Could you check a few things on this model? Use its own coordinates, in mm. A direction names the side the tool comes from. Coordinates: 2 decimals unless noted, no trailing zeros. Loops run counter-clockwise (first coordinate to the right, second up) from the corner with the lowest first, then second, coordinate; pieces in that order, holes last. Notation, with made-up numbers: M 74,5 L 79,5 A13 cw 79,19 Z; hole C 7.5,3.5 d6. An arc over 180 degrees is marked long. Write each question's results on one line, items separated by ' | '.
```python
from build123d import *

# Parameters (mm, degrees)
SKETCH_1_R                              = 38
SKETCH_1_R_2                            = 36
EXTRUDE_310_DEPTH                       = 15
EXTRUDE_START                           = -9
EXTRUDE_4_DEPTH                         = 9
FILLET_3_RADIUS                         = 5
FILLET_3_LENGTH                         = 9
PATTERN_CIRCULAR_4_COUNT                = 3
FILLET_3_OF_PATTERN_CIRCULAR_4_2_RADIUS = 5
FILLET_3_OF_PATTERN_CIRCULAR_4_2_LENGTH = 9
FILLET_3_OF_PATTERN_CIRCULAR_4_3_RADIUS = 5
FILLET_3_OF_PATTERN_CIRCULAR_4_3_LENGTH = 9
SKETCH_6_W                              = 176.950469939
SKETCH_6_H                              = 123.439451547
CUT_REVOLVE_861_ANGLE                   = 5
SKETCH_14_W                             = 84.084463922
SKETCH_14_H                             = 246.249240822
MM_7_D                                  = 5.2
MM_7_ON_FACE_2_D                        = 5.2
MM_7_ON_FACE_3_D                        = 5.2


with BuildPart() as part:
    # 草图1 → Extrude 310 (new body)
    with BuildSketch(Plane.XY):
        Circle(SKETCH_1_R)
        Circle(SKETCH_1_R_2, mode=Mode.SUBTRACT)
    extrude(amount=EXTRUDE_310_DEPTH)

    # 草图11 → 凸台-拉伸4 (add)
    with BuildSketch(Plane.XY.offset(15).offset(EXTRUDE_START)):
        with BuildLine():
            Line((-5, -37.669616404), (-5, -46.669616404))
            Line((-5, -46.669616404), (5, -46.669616404))
            Line((5, -46.669616404), (5, -37.669616404))
            ThreePointArc((5, -37.669616404), (0, -38), (-5, -37.669616404))
        make_face()
    extrude_4 = extrude(amount=EXTRUDE_4_DEPTH)

    # 圆角3: full round fillet: the end face becomes a half cylinder, R = half its width
    fillet_3_face = Plane((0, -46.669616404, 10.5), x_dir=(0, 0, 1), z_dir=(0, -1, 0))  # on the end face: x along it, z out of the body
    fillet_3_slab = fillet_3_face.offset(-FILLET_3_RADIUS / 2) * Box(FILLET_3_LENGTH, 2 * FILLET_3_RADIUS, FILLET_3_RADIUS, mode=Mode.PRIVATE)  # the body's end, R deep
    fillet_3_round = Plane((0, -41.669616404, 10.5), x_dir=(0, -1, 0), z_dir=(0, 0, 1)) * Cylinder(FILLET_3_RADIUS, FILLET_3_LENGTH, mode=Mode.PRIVATE)  # its axis R under the face
    add(fillet_3_slab - fillet_3_round, mode=Mode.SUBTRACT)

    # 阵列(圆周)4: 凸台-拉伸4 ×3 about axis
    pattern_circular_4_axis = Axis((0, 0, 0), (0, 0, 1))
    for i in range(1, PATTERN_CIRCULAR_4_COUNT):
        add(extrude_4.rotate(pattern_circular_4_axis, i * 360 / PATTERN_CIRCULAR_4_COUNT))

    # 圆角3 of Pattern Circular 4 2: full round fillet: the end face becomes a half cylinder, R = half its width
    fillet_3_of_pattern_circular_4_2_face = Plane((40.417073391, 23.334808202, 10.5), x_dir=(0, 0, 1), z_dir=(0.866025403784, 0.5, 0))  # on the end face: x along it, z out of the body
    fillet_3_of_pattern_circular_4_2_slab = fillet_3_of_pattern_circular_4_2_face.offset(-FILLET_3_OF_PATTERN_CIRCULAR_4_2_RADIUS / 2) * Box(FILLET_3_OF_PATTERN_CIRCULAR_4_2_LENGTH, 2 * FILLET_3_OF_PATTERN_CIRCULAR_4_2_RADIUS, FILLET_3_OF_PATTERN_CIRCULAR_4_2_RADIUS, mode=Mode.PRIVATE)  # the body's end, R deep
    fillet_3_of_pattern_circular_4_2_round = Plane((36.086946372, 20.834808202, 10.5), x_dir=(0.866025403784, 0.5, 0), z_dir=(0, 0, 1)) * Cylinder(FILLET_3_OF_PATTERN_CIRCULAR_4_2_RADIUS, FILLET_3_OF_PATTERN_CIRCULAR_4_2_LENGTH, mode=Mode.PRIVATE)  # its axis R under the face
    add(fillet_3_of_pattern_circular_4_2_slab - fillet_3_of_pattern_circular_4_2_round, mode=Mode.SUBTRACT)

    # 圆角3 of Pattern Circular 4 3: full round fillet: the end face becomes a half cylinder, R = half its width
    fillet_3_of_pattern_circular_4_3_face = Plane((-40.417073391, 23.334808202, 10.5), x_dir=(0, 0, 1), z_dir=(-0.866025403784, 0.5, 0))  # on the end face: x along it, z out of the body
    fillet_3_of_pattern_circular_4_3_slab = fillet_3_of_pattern_circular_4_3_face.offset(-FILLET_3_OF_PATTERN_CIRCULAR_4_3_RADIUS / 2) * Box(FILLET_3_OF_PATTERN_CIRCULAR_4_3_LENGTH, 2 * FILLET_3_OF_PATTERN_CIRCULAR_4_3_RADIUS, FILLET_3_OF_PATTERN_CIRCULAR_4_3_RADIUS, mode=Mode.PRIVATE)  # the body's end, R deep
    fillet_3_of_pattern_circular_4_3_round = Plane((-36.086946372, 20.834808202, 10.5), x_dir=(-0.866025403784, 0.5, 0), z_dir=(0, 0, 1)) * Cylinder(FILLET_3_OF_PATTERN_CIRCULAR_4_3_RADIUS, FILLET_3_OF_PATTERN_CIRCULAR_4_3_LENGTH, mode=Mode.PRIVATE)  # its axis R under the face
    add(fillet_3_of_pattern_circular_4_3_slab - fillet_3_of_pattern_circular_4_3_round, mode=Mode.SUBTRACT)

    # 草图6 → Cut-Revolve 861 (revolve, cut)
    with BuildSketch(Plane.XY):
        with Locations((-6.549725274, 19.685381772)):
            Rectangle(SKETCH_6_W, SKETCH_6_H)
    revolve(axis=Axis((41.8, -55, 0), (1, 0, 0)), revolution_arc=CUT_REVOLVE_861_ANGLE, mode=Mode.SUBTRACT)

    # 草图14 → Cut-Revolve 1016 (revolve, cut)
    with BuildSketch(Plane(origin=(0, 0, 0), x_dir=(0, 0, -1), z_dir=(1, 0, 0))):
        with Locations((-57.042231961, 14.211955097)):
            Rectangle(SKETCH_14_W, SKETCH_14_H)
    revolve(axis=Axis((0, 42.23348082, -180), (0, -1, 0)), mode=Mode.SUBTRACT)

    # 大小mm 暗销孔7 (through all)
    with Locations(Plane(origin=(-36.373066959, 21, 11.577660493), x_dir=(0.98244954099, 0, 0.186528548507), z_dir=(-0.186528548507, 0, 0.98244954099))):
        with Locations((0, 0)):
            Hole(MM_7_D / 2)

    # 大小mm 暗销孔7 on face 2 (through all)
    with Locations(Plane(origin=(0, -42, 15), x_dir=(1, 0, 0), z_dir=(0, 0, 1))):
        with Locations((0, 0)):
            Hole(MM_7_ON_FACE_2_D / 2)

    # 大小mm 暗销孔7 on face 3 (through all)
    with Locations(Plane(origin=(36.373066959, 21, 11.577660493), x_dir=(0.982449474222, 0, -0.186528900175), z_dir=(0.186528900175, 0, 0.982449474222))):
        with Locations((0, 0)):
            Hole(MM_7_ON_FACE_3_D / 2)


solid = part.part
```
(1) Imagine slicing it at D-D, the plane z = 9.5. State how many separate pieces and enclosed holes the cut face has, and give its area (3 significant figures).
Reported:
separate pieces: 1 | enclosed holes: 4 | area: 632 mm2
(2) Which directions (+Z, -Z, +X, -X, +Y, -Y) give clear straight access to the entire face, cutting with the end or side of a thin tool? Please do faces 1 (the flat face through (-5, -40, 10)), 2 (the flat face through (36.83, 15.49, 8.91)), 3 (the flat face through (-31.83, 24.15, 9.71)), 4 (the flat face through (-36.88, 15.52, 8.91)).
Reported:
face 1: +Z, -Z, -X, -Y | face 2: +Z, -Z, +X | face 3: +Z, -Z, +Y | face 4: +Z, -Z, -X
(3) If we mould it in two halves opening along X, with no side actions, what happens to faces 5 (the flat face through (5, -40, 10)), 6 (the cylindrical face through (-7.804, -35.144, 8.201)), 7 (the cylindrical face through (-0.11, -46.67, 10.56)), 8 (the flat face through (-0.19, 36.77, 8.03))? For each: released by +X, released by -X, zero draft, split by the parting line, or undercut.
Reported:
face 5: released by +X | face 6: undercut | face 7: split by the parting line | face 8: zero draft
(4) Will these pins go through, and if not, where does the flat tip stop? P1, Ø6, axis at y = -12, z = 6.5, coming from the -X side; P2, Ø2, axis at y = 16.5, z = 4.5, coming from the -X side; P3, Ø2.5, axis at x = 2, y = -41.5, coming from the -Z side; P4, Ø2, axis at y = -1.5, z = 8.5, coming from the +X side.
Reported:
P1: stops at x = -36.92 | P2: passes through | P3: stops at z = 6 | P4: stops at x = 38
(5) Please list where these lines run through material, in increasing order: probe 1 along Y at (x, z) = (0, 12); probe 2 along X at (y, z) = (0, 10); probe 3 along X at (y, z) = (-42, 12). Write a range as from..to.
Reported:
probe 1: y = -46.67..-44.6, -39.4..-36, 36..38 | probe 2: x = -38..-36, 36..38 | probe 3: x = -4.99..-2.6, 2.6..4.99
(6) Imagine slicing it at B-B, the plane x = 31.5. List the corners of the cut face in (y, z) for me, and give its area (3 significant figures).
Reported:
outline: M -21.25,2.95 L -17.43,3.29 L -17.43,12.44 L -21.25,12.44 Z; M 17.43,6.34 L 23.96,6.91 L 23.96,12.44 L 17.43,12.44 Z | area: 73.6 mm2
(7) Imagine slicing it at C-C, the plane x = 0. List the corners of the cut face in (y, z) for me, and give its area (3 significant figures).
Reported:
outline: M -46.67,6 L -44.6,6 L -44.6,15 L -46.67,15 Z; M -39.4,6 L -38,6 L -38,1.49 L -36,1.66 L -36,15 L -39.4,15 Z; M 36,7.96 L 38,8.14 L 38,15 L 36,15 Z | area: 72.0 mm2
(8) Imagine slicing it at A-A, the plane y = -30.5. List the corners of the cut face in (x, z) for me, and give its area (3 significant figures).
Reported:
outline: M -22.67,2.14 L -19.12,2.14 L -19.12,14.06 A195 ccw -22.67,13.68 Z; M 19.12,2.14 L 22.67,2.14 L 22.67,13.68 A195 ccw 19.12,14.06 Z | area: 83.1 mm2
